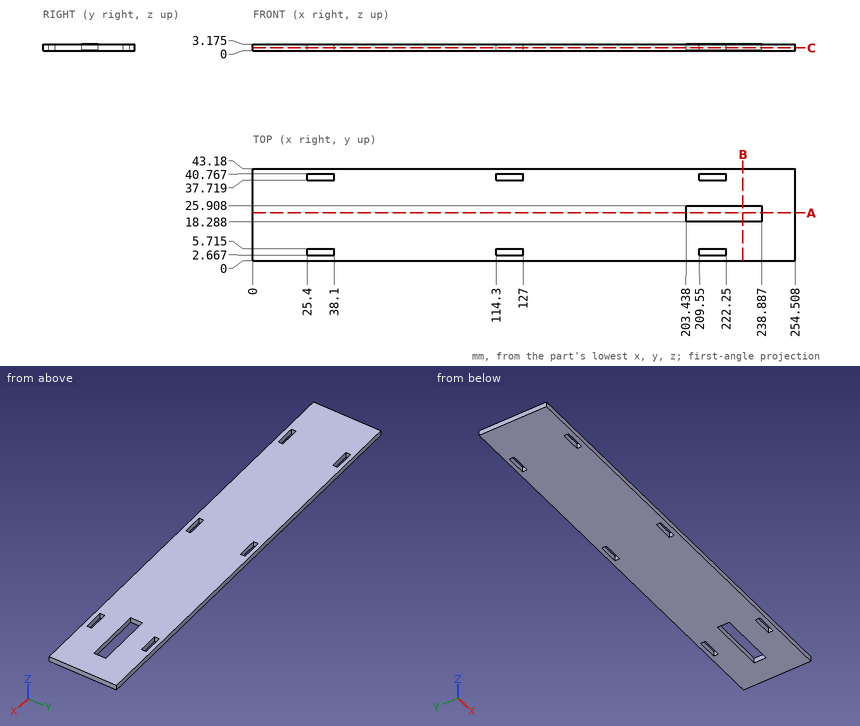
Design review of the part shown in the three views and the two pictorial views. Dimensions are in mm from the part's minimum x, y and z. Round coordinates to 2 decimals unless told otherwise and drop trailing zeros. Write each loop counter-clockwise with the first axis right and the second up, starting at its lowest first coordinate (ties: lowest second). Pieces come first, ordered by that corner, then holes. Notation, with made-up numbers: M 43,33.5 L 97,33.5 A31 cw 97,60.5 Z; hole C 59,43.25 d2. An arc over 180 degrees is marked long. One line per item, written item: value. Start each with the question number.
1. Take a section at B-B on x = 230. State the section outline as (y, z) points (3 decimals), then the cut area to 3 significant figures.
2. Take a section at A-A on y = 22.5. State the section outline as (x, z) points (1 decimal).
3. To check wall thickness, follow probe 1 along Y at (x, z) = (26, 2.45) (3 decimals); probe 2 along Y at (x, z) = (209, 0.1); probe 3 along X at (y, z) = (40.5, 1.25). State the ranges of each line that lie inside material, in increasing order. Write a range as from..to.
4. Take a section at C-C on z = 1.4. State how many separate pieces and enclosed holes the cut face has, then the cut area to 3 significant figures.
Computed:
1. outline: M 0,0 L 18.288,0 L 18.288,3.175 L 0,3.175 Z; M 25.908,0 L 43.18,0 L 43.18,3.175 L 25.908,3.175 Z
1. area: 113 mm²
2. outline: M 0,0 L 203.4,0 L 203.4,3.2 L 0,3.2 Z; M 238.9,0 L 254.5,0 L 254.5,3.2 L 238.9,3.2 Z
3. probe 1: y = 0..2.667, 5.715..37.719, 40.767..43.18
3. probe 2: y = 0..18.29, 25.91..43.18
3. probe 3: x = 0..25.4, 38.1..114.3, 127..209.55, 222.25..254.51
4. separate pieces: 1
4. enclosed holes: 7
4. area: 10,500 mm²
